```python
from build123d import *

# Parameters (mm, degrees)
F0_W     = 11
F0_H     = 15
F2_DEPTH = 20
F3_DEPTH = 19
F6_DEPTH = 15


with BuildPart() as f2:
    # F0 (on Top) → F2 (new body)
    with BuildSketch(Plane.XY):
        Rectangle(F0_W, F0_H)
    extrude(amount=F2_DEPTH)


with BuildPart() as f3:
    # F1 (on Top) → F3 (new body)
    with BuildSketch(Plane.XY):
        with BuildLine():
            ThreePointArc((9.9780160072, 0.6627190658), (-8.9648731573, -4.4306939945), (6.5869096361, 7.5241359269))
            Line((6.5869096361, 7.5241359269), (7.9042915633, 9.0289631123))
            ThreePointArc((7.9042915633, 9.0289631123), (-10.7578477888, -5.3168327934), (11.9736192086, 0.7952628789))
            Line((11.9736192086, 0.7952628789), (9.9780160072, 0.6627190658))
        make_face()
    extrude(amount=F3_DEPTH)


with BuildPart() as f6_tool:
    # F5 (on offset) → F6 (new body)
    with BuildSketch(Plane(origin=(-5.5, 0, 0), x_dir=(0, -1, 0), z_dir=(-1, 0, 0))):
        with BuildLine():
            ThreePointArc((0, 4), (2.4748737342, 5.0251262658), (3.5, 7.5))
            ThreePointArc((3.5, 7.5), (-2.4748737342, 9.9748737342), (0, 4))
        make_face()
    extrude(amount=-F6_DEPTH)


with BuildPart() as f2_1:
    add(f2.part)

    # F6: cut by f6_tool
    add(f6_tool.part, mode=Mode.SUBTRACT)


with BuildPart() as f3_1:
    add(f3.part)

    # F6: cut by f6_tool
    add(f6_tool.part, mode=Mode.SUBTRACT)


solid = f2_1.part
```
CAD build for the part. Positions are in the model's coordinates, mm. Give positions to 0.01 mm unless a question says otherwise; leave off trailing zeros. Loops run counter-clockwise (first coordinate to the right, second up) from the corner with the lowest first, then second, coordinate; pieces in that order, holes last. Notation, with made-up numbers: M 49.5,-5 L 66.5,-5 A16 cw 66.5,8 Z; hole C 78,-20.75 d11. An arc over 180 degrees is marked long. Use one line per item in the form item = value.
Item 1: Slice it at A-A (x = 1.25). List the corners of the cut face in (y, z).
Determined:
outline = M -7.5,0 L 7.5,0 L 7.5,20 L -7.5,20 Z; hole C 0,7.5 d7
Item 2: Drill centre lines: probe 1 along Y at (x, z) = (1, 7.5); probe 2 along Z at (x, y) = (-0.5, 0); probe 3 along Z at (x, y) = (-1, -2.25). Where is each one in solid material? Low to high. Write a range as from..to.
Determined:
probe_1 = -7.5..-3.5, 3.5..7.5
probe_2 = 0..4, 11..20
probe_3 = 0..4.82, 10.18..20
Item 3: Slice it at C-C (y = 2.5). List the corners of the cut face in (x, z).
Determined:
outline = M -5.5,0 L 5.5,0 L 5.5,5.05 L -5.5,5.05 Z; M -5.5,9.95 L 5.5,9.95 L 5.5,20 L -5.5,20 Z
Item 4: Slice it at B-B (z = 6.25). List the corners of the cut face in (x, y), plus the area to 3 significant figures.
Determined:
outline = M -5.5,-7.5 L 5.5,-7.5 L 5.5,-3.27 L -5.5,-3.27 Z; M -5.5,3.27 L 5.5,3.27 L 5.5,7.5 L -5.5,7.5 Z
area = 93.1 mm2
